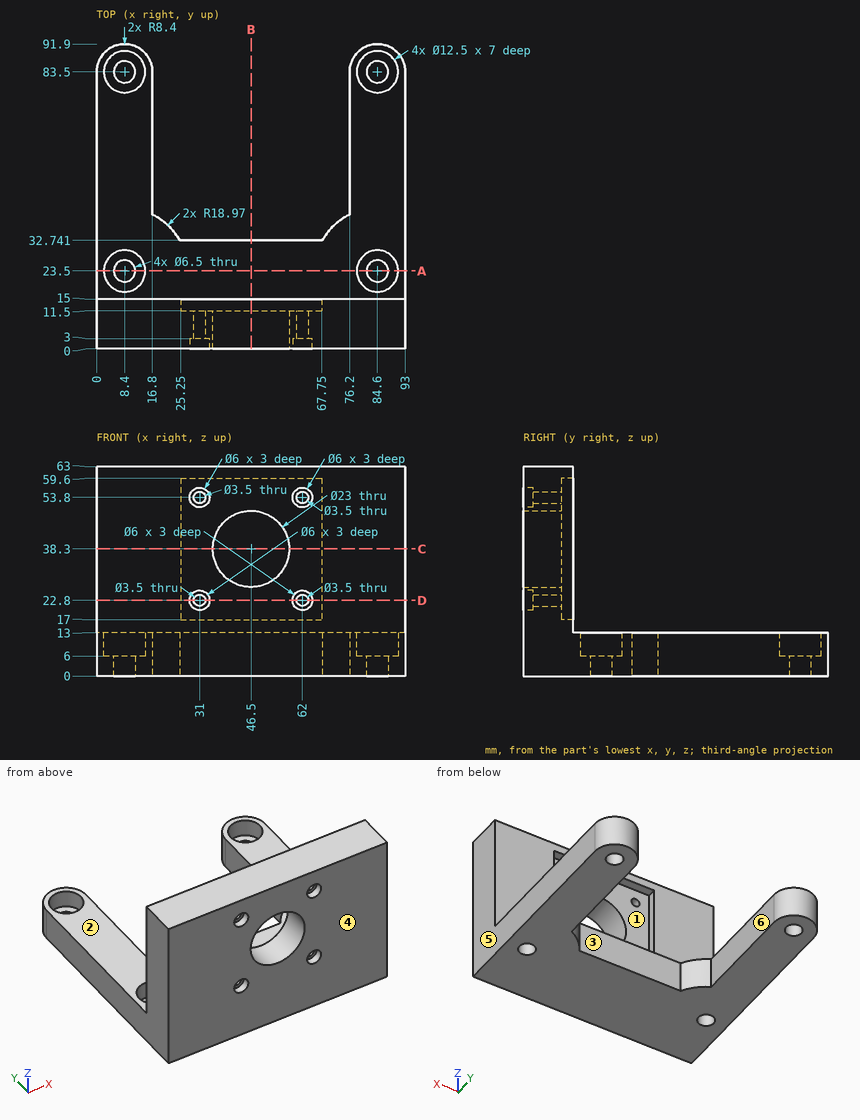
Geometry check sheet. Reference: drawing and pictorial views, mm from the part's lowest x, y, z. A direction names the side the tool comes from. Give positions to 0.01 mm unless a question says otherwise; leave off trailing zeros. Order: outer loops, then holes, each group sorted by start corner. A loop starts at its lowest first (then second) coordinate and runs counter-clockwise, first axis right, second up. Notation, with made-up numbers: M -30,59.5 L -8,59.5 A10 cw -8,67.5 Z; hole C 75.5,58.25 d9. An arc over 180 degrees is marked long. Use one line per item in the form item = value. Start each with the question number.
Q1. Scan lines: line 1 along Z through (x, y) = (31, 0.8); line 2 along Z through (x, y) = (62, 5.75); line 3 along X through (y, z) = (8.5, 22.8). Record each from-to range of solid material in increasing order. Write a range as [from, to].
Q2. Section check C-C (z = 38.3). Enter the section's corners in (x, y).
Q3. Mould release check, pull along X, two halves, no side actions. Record for the marked faces 4, 5 and 6: +X half, -X half, draft (parallel to the pull), parting line (faces both ways), or undercut.
Q4. Section check D-D (z = 22.8). Enter the section's corners in (x, y), then the cut area to 3 significant figures.
Q5. Section check B-B (x = 46.5). Enter the section's corners in (y, z).
Q6. Section check A-A (y = 23.5). Enter the section's corners in (x, z), then the cut area to 3 significant figures.
Q7. Access from +Z, -Z, +X, -X, +Y, -Y to the whole of each face (thin tool, end or side, straight path). Record for the marked faces 1, 2 and 3.
Q8. Go/stop test with flat-tipped pins: pin 1 Ø9.5 at (x, z) = (62, 22.8) entering from +Y; pin 2 Ø1.8 at (x, z) = (61.5, 55) entering from -Y; pin 3 Ø14.5 at (x, y) = (8.4, 83.5) entering from +Z; pin 4 Ø3 at (x, z) = (62, 53.8) entering from -Y. Record where each tip stops, or that it passes through.
Evaluation:
q1.line_1 = [0, 19.8], [25.8, 50.8], [56.8, 63]
q1.line_2 = [0, 21.05], [24.55, 52.05], [55.55, 63]
q1.line_3 = [0, 29.25], [32.75, 60.25], [63.75, 93]
q2.outline = M 0,0 L 35,0 L 35,11.5 L 25.25,11.5 L 25.25,15 L 0,15 Z; M 58,0 L 93,0 L 93,15 L 67.75,15 L 67.75,11.5 L 58,11.5 Z
q3.face_4 = draft
q3.face_5 = +X half
q3.face_6 = undercut
q4.outline = M 0,0 L 28,0 L 28,3 L 29.25,3 L 29.25,11.5 L 25.25,11.5 L 25.25,15 L 0,15 Z; M 32.75,3 L 34,3 L 34,0 L 59,0 L 59,3 L 60.25,3 L 60.25,11.5 L 32.75,11.5 Z; M 63.75,3 L 65,3 L 65,0 L 93,0 L 93,15 L 67.75,15 L 67.75,11.5 L 63.75,11.5 Z
q4.area = 1,150 mm2
q5.outline = M 0,0 L 32.74,0 L 32.74,13 L 15,13 L 15,17 L 11.5,17 L 11.5,26.8 L 0,26.8 Z; M 0,49.8 L 11.5,49.8 L 11.5,59.6 L 15,59.6 L 15,63 L 0,63 Z
q6.outline = M 0,0 L 5.15,0 L 5.15,6 L 2.15,6 L 2.15,13 L 0,13 Z; M 11.65,0 L 81.35,0 L 81.35,6 L 78.35,6 L 78.35,13 L 14.65,13 L 14.65,6 L 11.65,6 Z; M 87.85,0 L 93,0 L 93,13 L 90.85,13 L 90.85,6 L 87.85,6 Z
q6.area = 956 mm2
q7.face_1 = +Y
q7.face_2 = +Z, +X, -X, +Y
q7.face_3 = +Z, -Z, +Y
q8.pin_1 = 11.5
q8.pin_2 = 3
q8.pin_3 = 13
q8.pin_4 = through
